Build history of the part. All positions in model axes, mm. Face numbers are marked on the shaded views. A direction names the side the tool comes from. Give positions to 0.01 mm unless a question says otherwise; leave off trailing zeros. Loops run counter-clockwise (first coordinate to the right, second up) from the corner with the lowest first, then second, coordinate; pieces in that order, holes last. Notation, with made-up numbers: M 71,-32.5 L 109,-32.5 A24 ccw 109,-7.5 Z; hole C 47.25,86.5 d5. An arc over 180 degrees is marked long. Put each result on its own line as item: value.
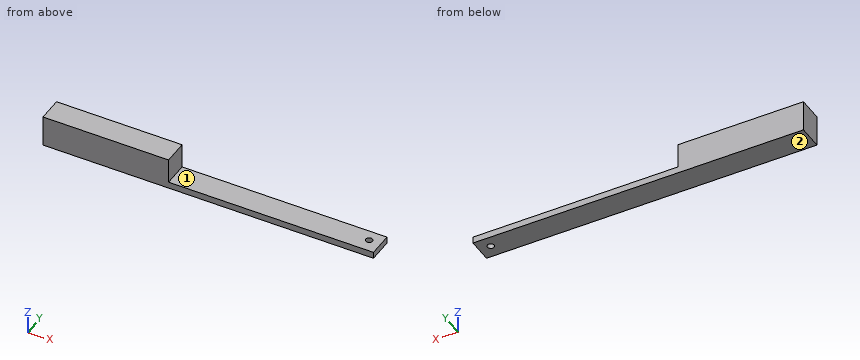
Autodesk Inventor part; units mm, degrees
ref_plane "YZ Plane" through (0, 0, 0) normal (1, 0, 0) x (0, 1, 0)
ref_plane "XZ Plane" through (0, 0, 0) normal (0, 1, 0) x (-1, 0, 0)
ref_plane "XY Plane" through (0, 0, 0) normal (0, 0, 1) x (1, 0, 0)
sketch "Эскиз1" plane through (0, 0, 0) normal (0, 0, 1) x (1, 0, 0)
  line L0 (0, 0) -> (200, 0)
  line L1 (200, 0) -> (200, 14.8438)
  line L2 (200, 14.8438) -> (0, 14.8438)
  line L3 (0, 14.8438) -> (0, 0)
  dimension "d2" = 200
extrude "Выдавливание1" add sketch "Эскиз1" along normal blind 4
sketch "Эскиз2" plane through (0, 0, 4) normal (0, 0, 1) x (1, 0, 0)
  line L0 (200, 14.8438) -> (0, 14.8438)
  line L1 (0, 0) -> (200, 0)
  line L2 (0, 14.8438) -> (76, 14.8438)
  line L3 (76, 14.8438) -> (76, 0)
  line L4 (76, 0) -> (0, 0)
  line L5 (0, 0) -> (0, 14.8438)
extrude "Выдавливание2" add sketch "Эскиз2" along normal blind 15
sketch "Эскиз3" plane through (0, 0, 4) normal (0, 0, 1) x (1, 0, 0)
  circle A0 centre (193, 8) radius 2
  point P0 (0, 0)
  dimension "d5" = 4
extrude "Выдавливание3" cut sketch "Эскиз3" against normal blind 10
properties part number "ведро 2 гол"
Q1. Tool access for the marked faces 1 and 2: list every direction of +Z, -Z, +X, -X, +Y, -Y with a clear straight run to the whole face (end or side of a thin tool).
Here are the results:
face 1: +Z, +X, +Y, -Y
face 2: -Z, +X, -X, +Y, -Y
Q2. Slice it at B-B (x = 193). List the corners of the cut face in (y, z), and give its area (3 significant figures).
Here are the results:
outline: M 0,0 L 6,0 L 6,4 L 0,4 Z; M 10,0 L 14.84,0 L 14.84,4 L 10,4 Z
area: 43.4 mm²
Q3. Probe line 1 (Y direction, x = 193, z = 0.95); line 2 (X direction, y = 12, z = 8); line 3 (Z direction, x = 186, y = 14). List the from-to ranges inside material, lowest first. Write a range as from..to.
Here are the results:
line 1: 0..6, 10..14.84
line 2: 0..76
line 3: 0..4
Q4. Slice it at C-C (z = 10.5). List the corners of the cut face in (x, y).
Here are the results:
outline: M 0,0 L 76,0 L 76,14.84 L 0,14.84 Z
Q5. Slice it at D-D (x = 79). List the corners of the cut face in (y, z).
Here are the results:
outline: M 0,0 L 14.84,0 L 14.84,4 L 0,4 Z
Q6. Drop flat-ended pins along their axis: pin 1 Ø4.5 at (y, z) = (4.5, 9) entering from +X; pin 2 Ø1 at (x, y) = (92, 3) entering from +Z; pin 3 Ø2 at (x, z) = (87, 5.5) entering from +Y. Give the stop position or say it passes through.
Here are the results:
pin 1: x = 76
pin 2: z = 4
pin 3: through
Q7. Slice it at A-A (y = 8). List the corners of the cut face in (x, z), and give its area (3 significant figures).
Here are the results:
outline: M 0,0 L 191,0 L 191,4 L 76,4 L 76,19 L 0,19 Z; M 195,0 L 200,0 L 200,4 L 195,4 Z
area: 1,920 mm²
